```python
from build123d import *

# Parameters (mm, degrees)
BOSS_EXTRUDE2_DEPTH = 5


with BuildPart() as part:
    # Sketch1 → Boss-Extrude2 (new body)
    with BuildSketch(Plane.XY):
        Polygon((0, 0), (15, 0), (15, -5), (25, -5), (25, 0), (35, 0), (35, -5), (45, -5), (45, 0), (55, 0), (55, -5), (65, -5), (65, 0), (75, 0), (75, -5), (85, -5), (85, 0), (95, 0), (95, -5), (105, -5), (105, 0), (115, 0), (115, -5), (125, -5), (125, 0), (135, 0), (135, -5), (145, -5), (145, 0), (155, 0), (155, -5), (165, -5), (165, 0), (180, 0), (180, 50), (165, 50), (165, 55), (155, 55), (155, 50), (145, 50), (145, 55), (135, 55), (135, 50), (125, 50), (125, 55), (115, 55), (115, 50), (105, 50), (105, 55), (95, 55), (95, 50), (85, 50), (85, 55), (75, 55), (75, 50), (65, 50), (65, 55), (55, 55), (55, 50), (45, 50), (45, 55), (35, 55), (35, 50), (25, 50), (25, 55), (15, 55), (15, 50), (0, 50), align=None)
    extrude(amount=BOSS_EXTRUDE2_DEPTH)


solid = part.part
```
Geometry: final body of the model. Coordinates: model frame, mm. A direction names the side the tool comes from. Round coordinates to 2 decimals unless told otherwise and drop trailing zeros. Write each loop counter-clockwise with the first axis right and the second up, starting at its lowest first coordinate (ties: lowest second). Pieces come first, ordered by that corner, then holes. Notation, with made-up numbers: M 31.5,-5.5 L 37.5,-5.5 A22 cw 37.5,12.5 Z; hole C 70.25,61.5 d1. An arc over 180 degrees is marked long. Answer in a Markdown table with one row per item. Add a question column.
(1) Draft query along X for faces 6 (the face through (20, -5, 2)), 7 (the face through (180, 25, 2)), 8 (the face through (25, 52, 2)). Return one class per face: pulls with the +X half, pulls with the -X half, needs draft (parallel to the pull), parting line crosses it, or undercut.
(2) Cut plane A-A, the plane x = 147.5. Return the cut outline in (y, z).
(3) Reachability of faces 1 (the face through (173, 50, 2)), 2 (the face through (60, 55, 2)), 3 (the face through (110, 50, 2)), 4 (the face through (130, 0, 2)), 5 (the face through (172, 0, 2)) from +Z, -Z, +X, -X, +Y, -Y: full face, straight path, thin tool, end or side. Return the list, or none.
(4) Contact query for flat-ended pins moving along their axis: pin 1 (2.5 mm diameter, centred on x = 173.5, z = 3, fed in from -Y); pin 2 (3 mm diameter, centred on y = 38, z = 0.5, fed in from -X); pin 3 (2.5 mm diameter, centred on x = 150, z = 3, fed in from +Y); pin 4 (1.5 mm diameter, centred on y = -3, z = 1.5, fed in from +X). Output: stop coordinate, or through.
(5) Ray query, L1, parallel to Y at x = 9.5, z = 2.45. Return the intervals inside material, ascending.
Established:
| question | item | result |
|---|---|---|
| 1 | face 6 | needs draft |
| 1 | face 7 | pulls with the +X half |
| 1 | face 8 | undercut |
| 2 | outline | M 0,0 L 50,0 L 50,5 L 0,5 Z |
| 3 | face 1 | +Z, -Z, +X, +Y |
| 3 | face 2 | +Z, -Z, +X, -X, +Y |
| 3 | face 3 | +Z, -Z, +Y |
| 3 | face 4 | +Z, -Z, -Y |
| 3 | face 5 | +Z, -Z, +X, -Y |
| 4 | pin 1 | y = 0 |
| 4 | pin 2 | x = 0 |
| 4 | pin 3 | y = 50 |
| 4 | pin 4 | x = 165 |
| 5 | L1 | 0 to 50 |
